Read the model definition and answer for the solid it produces. Units are mm, in the model's axes. Give positions to 0.01 mm unless a question says otherwise; leave off trailing zeros. Loops run counter-clockwise (first coordinate to the right, second up) from the corner with the lowest first, then second, coordinate; pieces in that order, holes last. Notation, with made-up numbers: (-12.5, 74) - (21.5, 74) arc R26 cw to (21.5, 111) - close; hole circle Ø7 at (43, 24.25). An arc over 180 degrees is marked (long way). Put each result on its own line as item: value. Start each with the question number.
1. Consider L1, parallel to Y at x = 6.75, z = 0; L2, parallel to Y at x = 2.25, z = -2.5; L3, parallel to Z at x = 4.5, y = -25. Determine where each line is inside the solid, lowest interval first. Write a range as from..to.
2. A cutting plane is placed at C-C, the plane z = 0. Determine the outline of the cut face in (x, y), plus the area to 3 significant figures.
3. A cutting plane is placed at D-D, the plane y = -25. Determine the outline of the cut face in (x, z), plus the area to 3 significant figures.
4. A cutting plane is placed at B-B, the plane x = 2.5. Determine the outline of the cut face in (y, z).
5. Given pin 1 Ø2 at (x, z) = (4.5, -38) entering from -Y; pin 2 Ø2 at (x, z) = (7.5, -9) entering from -Y; pin 3 Ø1.5 at (x, z) = (5.5, -29.5) entering from +Y, each flat-ended and moving along its own axis, determine where each tip first touches the part or whether it passes through.
6. A cutting plane is placed at A-A, the plane y = 0. Determine the outline of the cut face in (x, z), plus the area to 3 significant figures.
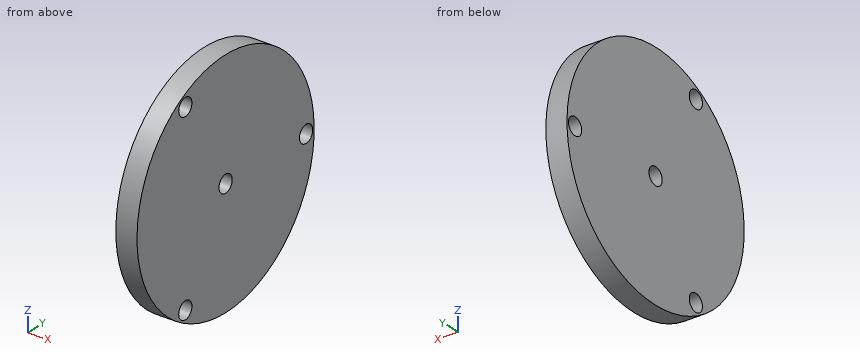
```python
from build123d import *

# Parameters (mm, degrees)
SKETCH1_R           = 55
BOSS_EXTRUDE1_DEPTH = 10
SKETCH2_R           = 4.1
CUT_EXTRUDE1_DEPTH  = 79.421935707


with BuildPart() as part:
    # Sketch1 → Boss-Extrude1 (new body)
    with BuildSketch(Plane(origin=(0, 0, 0), x_dir=(0, 0, -1), z_dir=(1, 0, 0))):
        Circle(SKETCH1_R)
    extrude(amount=BOSS_EXTRUDE1_DEPTH)

    # Sketch2 → Cut-Extrude1 (cut, through all)
    with BuildSketch(Plane(origin=(0, 0, 0), x_dir=(0, 0, -1), z_dir=(1, 0, 0))):
        Circle(SKETCH2_R)
        with Locations((0, 50)):
            Circle(SKETCH2_R)
        with Locations((43.301270189, -25)):
            Circle(SKETCH2_R)
        with Locations((-43.301270189, -25)):
            Circle(SKETCH2_R)
    extrude(amount=CUT_EXTRUDE1_DEPTH, mode=Mode.SUBTRACT)


solid = part.part
```
Return value:
1. L1: y = -55..-4.1, 4.1..45.9, 54.1..55
1. L2: y = -54.94..-3.25, 3.25..46.75, 53.25..54.94
1. L3: z = -48.99..-47.4, -39.2..39.2, 47.4..48.99
2. outline: (0, -55) - (10, -55) - (10, -4.1) - (0, -4.1) - close; (0, 4.1) - (10, 4.1) - (10, 45.9) - (0, 45.9) - close; (0, 54.1) - (10, 54.1) - (10, 55) - (0, 55) - close
2. area: 936 mm2
3. outline: (0, -48.99) - (10, -48.99) - (10, -47.4) - (0, -47.4) - close; (0, -39.2) - (10, -39.2) - (10, 39.2) - (0, 39.2) - close; (0, 47.4) - (10, 47.4) - (10, 48.99) - (0, 48.99) - close
3. area: 816 mm2
4. outline: circle Ø110 at (0, 0); hole circle Ø8.2 at (-25, -43.3); hole circle Ø8.2 at (-25, 43.3); hole circle Ø8.2 at (0, 0); hole circle Ø8.2 at (50, 0)
5. pin 1: stops at y = -40.69
5. pin 2: stops at y = -54.42
5. pin 3: stops at y = 46.89
6. outline: (0, -55) - (10, -55) - (10, -4.1) - (0, -4.1) - close; (0, 4.1) - (10, 4.1) - (10, 55) - (0, 55) - close
6. area: 1,020 mm2
